Verification items for the finished model (mm, model axes). A direction names the side the tool comes from. Round coordinates to 2 decimals unless told otherwise and drop trailing zeros. Write each loop counter-clockwise with the first axis right and the second up, starting at its lowest first coordinate (ties: lowest second). Pieces come first, ordered by that corner, then holes. Notation, with made-up numbers: (34, 85) - (44, 85) arc R14 cw to (44, 102) - close; hole circle Ø10 at (9.25, 63.5). An arc over 180 degrees is marked (long way). Answer as a JSON object with one key per item and string values. Group by question number.
1) Mould release check, pull along Y, two halves, no side actions. Record for faces 1 (the cylindrical face through (-105.55, 36.93, 5.07)), 2 (the conical face through (-15.695, 25.263, 5.053)), 3 (the flat face through (-54, 19, 10)), 4 (the cylindrical face through (-7.605, 26.867, 5.303)): +Y half, -Y half, draft (parallel to the pull), parting line (faces both ways), or undercut.
2) Go/stop test with flat-tipped pins: pin 1 Ø2 at (x, z) = (-22, 15) entering from -Y; pin 2 Ø3 at (x, z) = (-2.4, 12.4) entering from +Y; pin 3 Ø12 at (x, y) = (-67, 8) entering from +Z; pin 4 Ø3.5 at (x, y) = (-10.5, 4.5) entering from -Z. Record where each tip stops, or that it passes through.
3) Section check B-B (x = -99). Enter the section's corners in (y, z).
4) Section check D-D (z = 23.5). Enter the section's corners in (x, y), then the cut area to 3 significant figures.
5) Thickness scan on line 1 (Y direction, x = -14, z = 5); line 2 (Y direction, x = -99, z = 3); line 3 (X direction, y = 5, z = 2). Record the ranges inside material, lowest first.
6) Set-up check for faces 5 (the flat face through (-22, 10, 18)), 6 (the cylindrical face through (-13.814, 6.804, 3.819)), 7 (the cylindrical face through (-2.67, 5.07, 29.02)): record each of +Z, -Z, +X, -X, +Y, -Y from which the full face is reachable in a straight line by a thin tool's end or side.
7) Section check A-A (y = 32.01). Enter the section's corners in (x, z), then the cut area to 3 significant figures.
8) Section check C-C (z = 2). Enter the section's corners in (x, y), then the cut area to 3 significant figures.
Autodesk Inventor part; units mm, degrees
ref_plane "YZ Plane" through (0, 0, 0) normal (1, 0, 0) x (0, 1, 0)
ref_plane "XZ Plane" through (0, 0, 0) normal (0, 1, 0) x (-1, 0, 0)
ref_plane "XY Plane" through (0, 0, 0) normal (0, 0, 1) x (1, 0, 0)
ref_plane "Arbeitsebene1" through (0, 0, 0) normal (0, 0, 1) x (1, 0, 0)
sketch "Skizze1" plane through (0, 0, 0) normal (0, 0, 1) x (1, 0, 0)
  line L0 (-106.15, 0) -> (-106.15, 8)
  line L1 (0, 0) -> (-106.15, 0)
  line L2 (0, 0) -> (0, 37.5)
  line L3 (0, 37.5) -> (-176.65, 37.5)
  line L4 (-176.65, 0) -> (-176.65, 37.5)
  line L5 (-137.15, 0) -> (-176.65, 0)
  line L6 (-137.15, 8) -> (-137.15, 0)
  arc A0 (-135.15, 10) -> (-137.15, 8) centre (-135.15, 8) ccw
  line L7 (-108.15, 10) -> (-135.15, 10)
  arc A1 (-106.15, 8) -> (-108.15, 10) centre (-108.15, 8) ccw
  circle A2 centre (-99, 32.01) radius 1.9 construction
  arc A3 (-9.5, 2.18) -> (-9.5, 9.18) centre (-9.5, 5.68) ccw
  line L8 (-10.5, 2.18) -> (-9.5, 2.18)
  arc A4 (-10.5, 9.18) -> (-10.5, 2.18) centre (-10.5, 5.68) ccw
  line L9 (-9.5, 9.18) -> (-10.5, 9.18)
  circle A5 centre (-99, 5.68) radius 1.525 construction
  circle A6 centre (-99, 32.01) radius 1.4
  circle A7 centre (-99, 5.68) radius 1.4
  line L10 (-20.2, 0) -> (-20.2, -25.9)
  line L11 (0, 0) -> (0, -25.9)
  line L12 (-106.15, 37.5) -> (0, 37.5)
  line L13 (0, 37.5) -> (0, 0)
  line L14 (0, 0) -> (-106.15, 0)
  line L15 (-106.15, 0) -> (-106.15, 37.5)
  dimension "d0" = 2.8
  dimension "d1" = 2.8
extrude "Extrusion1" add sketch "Skizze1" along normal blind 10 contours L0 L15 L3 L2 L1
ref_plane "Arbeitsebene2" through (0, 0, 25.2) normal (0, 1, 0) x (0, 0, -1)
sketch "Skizze2" plane through (0, 0, 25.2) normal (0, 1, 0) x (0, 0, -1)
  line L0 (-5, 17.9) -> (-5, 2.3)
  arc A0 (-5, 2.3) -> (-2.7, 0) centre (-2.7, 2.3) ccw
  line L1 (-2.7, 0) -> (12.9, 0)
  arc A1 (12.9, 0) -> (15.2, 2.3) centre (12.9, 2.3) ccw
  line L2 (15.2, 2.3) -> (15.2, 17.9)
  arc A2 (15.2, 17.9) -> (12.9, 20.2) centre (12.9, 17.9) ccw
  line L3 (12.9, 20.2) -> (-2.7, 20.2)
  arc A3 (-2.7, 20.2) -> (-5, 17.9) centre (-2.7, 17.9) ccw
  circle A4 centre (5.1, 10.1) radius 8
  circle A5 centre (-2.6, 2.4) radius 1
  circle A6 centre (12.8, 2.4) radius 1
  circle A7 centre (12.8, 17.8) radius 1
  circle A8 centre (-2.6, 17.8) radius 1
  line L4 (-5, 17.9) -> (-5, 22.9389)
  line L5 (-5, 22.9389) -> (15.2, 43.1389)
  line L6 (15.2, 106.15) -> (15.2, 0)
  line L7 (15.2, 0) -> (15.2, 2.3)
  line L8 (15.2, 0) -> (-5, 0)
  line L9 (-5, 0) -> (-5, 20.2)
  line L10 (-5, 20.2) -> (15.2, 20.2)
  line L11 (15.2, 20.2) -> (15.2, 0)
  point P0 (25.2, 0)
  point P1 (15.2, 20.2)
  point P2 (15.2, 17.9)
  point P3 (12.9, 0)
  point P4 (15.2, 2.3)
  dimension "d13" = 135
extrude "Extrusion2" add sketch "Skizze2" along normal blind 10 contours A3 L3 A2 L2 A1 L1 A0 L0 | L4 L10 A3 | L10 L4 L5 L6 L3 | L10 L6 A2 | A1 L6 L8
sketch "Skizze3" plane through (-106.15, 37.5, 0) normal (0, 1, 0) x (1, 0, 0)
  circle A0 centre (96.05, -20.1) radius 8
  circle A1 centre (88.35, -27.8) radius 1
  circle A2 centre (88.35, -12.4) radius 1
  circle A3 centre (103.75, -27.8) radius 1
  circle A4 centre (103.75, -12.4) radius 1
  circle A5 centre (96.05, -20.1) radius 9
  circle A6 centre (88.35, -27.8) radius 1.25
  circle A7 centre (103.75, -27.8) radius 1.25
  circle A8 centre (103.75, -12.4) radius 1.25
  circle A9 centre (88.35, -12.4) radius 1.25
  point P0 (106.15, 0)
  point P1 (102.2136, -10)
  point P2 (89.8864, -10)
  dimension "d6" = 18
  dimension "d7" = 2.5
  dimension "d8" = 2.5
  dimension "d9" = 2.5
  dimension "d10" = 2.5
extrude "Extrusion3" cut sketch "Skizze3" against normal through all contours A0 | A1 | A2 | A3 | A4 | A5 | A6 | A7 | A8 | A9
fillet "Rundung1" radius 2 4 edges at (-22.9389, 5, 30.2) (-43.1389, 5, 10) (-106.15, 37.5, 5) (-106.15, 0, 5)
sketch "Skizze4" plane through (0, 0, 0) normal (1, 0, 0) x (0, 0, -1)
  circle A0 centre (-5, 25.5) radius 1.75
  circle A1 centre (-5, 5.5) radius 1.75
  point P0 (0, 0)
hole "Bohrung1" at (0, 25.5, 5) at (0, 5.5, 5) direction (-1, 0, 0) diameter 2.8 depth 15 tip angle 118
sketch "Skizze5" plane through (0, 0, 10) normal (0, 0, 1) x (1, 0, 0)
  arc A0 (-106.15, 2) -> (-104.15, 0) centre (-104.15, 2) ccw
  line L0 (-104.15, 0) -> (-43.9674, 0)
  line L1 (-43.9674, 10) -> (-43.9674, 0)
  line L2 (-43.9674, 10) -> (0, 10)
  line L3 (0, 10) -> (0, 37.5)
  line L4 (0, 37.5) -> (-104.15, 37.5)
  arc A1 (-104.15, 37.5) -> (-106.15, 35.5) centre (-104.15, 35.5) ccw
  line L5 (-106.15, 35.5) -> (-106.15, 2)
  circle A2 centre (-99, 32.01) radius 1.4
  circle A3 centre (-99, 5.68) radius 1.4
  point P0 (0, 0)
hole "Bohrung2" at (-99, 5.68, 10) at (-99, 32.01, 10) direction (0, 0, -1) diameter 4 depth 15 tip angle 118
properties part number "OT2-Gripper_base"
Returned:
{
 "1": {"face 1": "+Y half", "face 2": "undercut", "face 3": "draft", "face 4": "undercut"},
 "2": {"pin 1": "y = 0", "pin 2": "y = 10", "pin 3": "z = 10", "pin 4": "z = 10"},
 "3": {"outline": "(0, 0) - (3.68, 0) - (3.68, 10) - (0, 10) - close; (7.68, 0) - (30.01, 0) - (30.01, 10) - (7.68, 10) - close; (34.01, 0) - (37.5, 0) - (37.5, 10) - (34.01, 10) - close"},
 "4": {"outline": "(-29.64, 0) - (-18.43, 0) - (-18.43, 10) - (-29.64, 10) - close; (-1.77, 0) - (0, 0) - (0, 10) - (-1.77, 10) - close", "area": "130 mm2"},
 "5": {"line 1": "0 to 4.1, 6.9 to 24.1, 26.9 to 37.5", "line 2": "0 to 3.68, 7.68 to 30.01, 34.01 to 37.5", "line 3": "-106.15 to -100.88, -97.12 to -13.93, -6.07 to 0"},
 "6": {"face 5": "+Z, +X, -X, +Y", "face 6": "-Z", "face 7": "+Y, -Y"},
 "7": {"outline": "(-106.15, 0) - (-101, 0) - (-101, 10) - (-106.15, 10) - close; (-97, 0) - (0, 0) - (0, 10) - (-97, 10) - close", "area": "1,020 mm2"},
 "8": {"outline": "(-106.15, 2) arc R2 ccw to (-104.15, 0) - (0, 0) - (0, 37.5) - (-104.15, 37.5) arc R2 ccw to (-106.15, 35.5) - close; hole circle Ø4 at (-99, 5.68); hole circle Ø4 at (-99, 32.01); hole (-10.5, 2.18) - (-9.5, 2.18) arc R3.5 ccw to (-9.5, 9.18) - (-10.5, 9.18) arc R3.5 ccw to start", "area": "3,910 mm2"}
}
